from build123d import *
from build123d.topology import SkipClean

# Parameters (mm, degrees)
BOSS_EXTRUDE1_START     = 3
SKETCH1_W               = 130
SKETCH1_H               = 16
BOSS_EXTRUDE1_DEPTH     = 6
BOSS_EXTRUDE2_START     = 3
SKETCH2_R               = 12
BOSS_EXTRUDE2_DEPTH     = 6
BOSS_EXTRUDE3_START     = 3
SKETCH3_R               = 14
BOSS_EXTRUDE3_DEPTH     = 6
BOSS_EXTRUDE4_START     = 2.5
SKETCH4_R               = 14
BOSS_EXTRUDE4_DEPTH     = 8
CUT_EXTRUDE1_DEPTH      = 146.059470563
CUT_EXTRUDE1_DEPTH_BACK = 146.059470563
SKETCH5_R               = 3.25
CUT_EXTRUDE2_DEPTH      = 146.059470563
CUT_EXTRUDE2_DEPTH_BACK = 146.059470563
SKETCH6_R               = 1.725
CUT_EXTRUDE3_START      = 3
SKETCH7_R               = 2.9
CUT_EXTRUDE3_DEPTH      = 2.2
CUT_EXTRUDE4_START      = 3
SKETCH8_R               = 2.9
CUT_EXTRUDE4_DEPTH      = 2.2
CUT_EXTRUDE5_START      = 3.5
SKETCH9_R               = 11
CUT_EXTRUDE5_DEPTH      = 7
CUT_EXTRUDE6_DEPTH      = 146.059470563
CUT_EXTRUDE6_DEPTH_BACK = 146.059470563
SKETCH10_R              = 8


with BuildPart() as part:
    # Sketch1 → Boss-Extrude1 (new body)
    with BuildSketch(Plane.XY.offset(BOSS_EXTRUDE1_START)):
        with Locations((65, 0)):
            Rectangle(SKETCH1_W, SKETCH1_H)
    extrude(amount=BOSS_EXTRUDE1_DEPTH)

    # Sketch2 → Boss-Extrude2 (add)
    with BuildSketch(Plane.XY.offset(BOSS_EXTRUDE2_START)):
        Circle(SKETCH2_R)
    extrude(amount=BOSS_EXTRUDE2_DEPTH)

    # Sketch3 → Boss-Extrude3 (add)
    with BuildSketch(Plane.XY.offset(BOSS_EXTRUDE3_START)):
        with Locations((130, 0)):
            Circle(SKETCH3_R)
    extrude(amount=BOSS_EXTRUDE3_DEPTH)

    # Sketch4 → Boss-Extrude4 (add)
    with SkipClean():  # the faces are left unmerged after this step: merging them gives an invalid solid
        with BuildSketch(Plane.XY.offset(BOSS_EXTRUDE4_START)):
            with Locations((130, 0)):
                Circle(SKETCH4_R)
        extrude(amount=BOSS_EXTRUDE4_DEPTH)
    add(part.part.scale(1), mode=Mode.REPLACE)  # the faces are merged on a copy

    # Sketch5 → Cut-Extrude1 (cut, two sides: drawn at the far end of the back side and taken through both)
    with BuildSketch(Plane.XY.offset(-CUT_EXTRUDE1_DEPTH_BACK)):
        Circle(SKETCH5_R)
    extrude(amount=CUT_EXTRUDE1_DEPTH + CUT_EXTRUDE1_DEPTH_BACK, mode=Mode.SUBTRACT)

    # Sketch6 → Cut-Extrude2 (cut, two sides: drawn at the far end of the back side and taken through both)
    with BuildSketch(Plane.XY.offset(-CUT_EXTRUDE2_DEPTH_BACK)):
        with Locations((8, 0)):
            Circle(SKETCH6_R)
        with Locations((20, 0)):
            Circle(SKETCH6_R)
    extrude(amount=CUT_EXTRUDE2_DEPTH + CUT_EXTRUDE2_DEPTH_BACK, mode=Mode.SUBTRACT)

    # Sketch7 → Cut-Extrude3 (cut)
    with BuildSketch(Plane.XY.offset(CUT_EXTRUDE3_START)):
        with Locations((8, 0)):
            Circle(SKETCH7_R)
    extrude(amount=CUT_EXTRUDE3_DEPTH, mode=Mode.SUBTRACT)

    # Sketch8 → Cut-Extrude4 (cut)
    with BuildSketch(Plane.XY.offset(CUT_EXTRUDE4_START)):
        with Locations((20, 0)):
            Circle(SKETCH8_R)
    extrude(amount=CUT_EXTRUDE4_DEPTH, mode=Mode.SUBTRACT)

    # Sketch9 → Cut-Extrude5 (cut)
    with BuildSketch(Plane.XY.offset(CUT_EXTRUDE5_START)):
        with Locations((130, 0)):
            Circle(SKETCH9_R)
    extrude(amount=CUT_EXTRUDE5_DEPTH, mode=Mode.SUBTRACT)

    # Sketch10 → Cut-Extrude6 (cut, two sides: drawn at the far end of the back side and taken through both)
    with BuildSketch(Plane.XY.offset(-CUT_EXTRUDE6_DEPTH_BACK)):
        with Locations((130, 0)):
            Circle(SKETCH10_R)
    extrude(amount=CUT_EXTRUDE6_DEPTH + CUT_EXTRUDE6_DEPTH_BACK, mode=Mode.SUBTRACT)


solid = part.part
Design review of the part built by this model. Coordinates are the model's own, in mm. A direction names the side the tool comes from. Give positions to 0.01 mm unless a question says otherwise; leave off trailing zeros. Loops run counter-clockwise (first coordinate to the right, second up) from the corner with the lowest first, then second, coordinate; pieces in that order, holes last. Notation, with made-up numbers: M 44.25,54.25 L 59.25,54.25 A22 ccw 59.25,77.25 Z; hole C 78,63.5 d1. An arc over 180 degrees is marked long. Write item = value, one per line.
Q1. We need section D-D (y = 0). Count the separate pieces of the cut face and the enclosed holes in it, plus the area to 3 significant figures.
Output values:
separate_pieces = 5
enclosed_holes = 0
area = 731 mm^2
Q2. Insertion check: pin 1 (2 mm diameter, centred on y = -6, z = 7.5, fed in from +X); pin 2 (6.5 mm diameter, centred on x = 7, y = 0, fed in from -Z); pin 3 (3 mm diameter, centred on x = 94.5, z = 3.5, fed in from +Y). Each pin has a flat end and moves straight along its axis. Give the tip position at first contact, or say it passes through.
Output values:
pin_1 = 143.08
pin_2 = 3
pin_3 = 8
Q3. We need section B-B (y = -9.5). Give the boundary of the cut face in (x, z).
Output values:
outline = M -7.33,3 L 7.33,3 L 7.33,9 L -7.33,9 Z; M 119.72,2.5 L 140.28,2.5 L 140.28,10.5 L 135.55,10.5 L 135.55,3.5 L 124.45,3.5 L 124.45,10.5 L 119.72,10.5 Z
Q4. We need section A-A (x = 0). Give the boundary of the cut face in (y, z), plus the area to 3 significant figures.
Output values:
outline = M -12,3 L -3.25,3 L -3.25,9 L -12,9 Z; M 3.25,3 L 12,3 L 12,9 L 3.25,9 Z
area = 105 mm^2
Q5. For faces 4 (the flat face through (22, 0, 5.2)), 5 (the flat face through (128, -8, 3.5)), 6 (the flat face through (63, -8, 6)), list the 3-axis set-ups (+Z, -Z, +X, -X, +Y, -Y) from which the entire face can be reached by the end or side of a thin tool; tool diameter is ignored.
Output values:
face_4 = -Z
face_5 = +Z
face_6 = +Z, -Z, -Y
Q6. Draft analysis for pull direction Y (two halves, no side actions). For faces 1 (the cylindrical face through (-12, 0, 6)), 2 (the flat face through (136, -6, 2.5)), 3 (the cylindrical face through (5.1, 0.1, 4.1)), state which applies: +Y half, -Y half, draft (parallel to the pull), parting line (faces both ways), or undercut.
Output values:
face_1 = parting line
face_2 = draft
face_3 = undercut
Q7. We need section C-C (x = 20). Give the boundary of the cut face in (y, z) (3 decimals), plus the area to 3 significant figures.
Output values:
outline = M -8,3 L -2.9,3 L -2.9,5.2 L -1.725,5.2 L -1.725,9 L -8,9 Z; M 1.725,5.2 L 2.9,5.2 L 2.9,3 L 8,3 L 8,9 L 1.725,9 Z
area = 70.1 mm^2
Q8. To check wall thickness, follow line 1 (Y direction, x = 130, z = 3.2); line 2 (Y direction, x = 0, z = 5.1); line 3 (X direction, y = 0, z = 2.75). State the ranges of each line that lie inside material, in increasing order. Write a range as [from, to].
Output values:
line_1 = [-14, -8], [8, 14]
line_2 = [-12, -3.25], [3.25, 12]
line_3 = [116, 122], [138, 144]
